Part model, mm, in its own coordinate system. Face numbers are marked on the shaded views. A direction names the side the tool comes from. Round coordinates to 2 decimals unless told otherwise and drop trailing zeros. Write each loop counter-clockwise with the first axis right and the second up, starting at its lowest first coordinate (ties: lowest second). Pieces come first, ordered by that corner, then holes. Notation, with made-up numbers: M -21.75,32 L 37.25,32 A28 ccw 37.25,63 Z; hole C 11,-0.5 d1. An arc over 180 degrees is marked long. Use a Markdown table: item, result. Add a question column.
1) Slice it at A-A on y = 13.5. Write the cut outline in (x, z), plus the area to 3 significant figures.
2) Wall check: probe 1 along X at (y, z) = (13.5, 5.8); probe 2 along X at (y, z) = (13.5, 3.3); probe 3 along X at (y, z) = (7.5, 5.75). Give the ranges that are in metal, low to high.
3) Slice it at D-D on y = 8.5. Write the cut outline in (x, z).
4) Slice it at C-C on z = 1. Write the cut outline in (x, y), plus the area to 3 significant figures.
5) Which spindle directions (+Z, -Z, +X, -X, +Y, -Y) get a long thin tool onto all of the face, cutting with end or side? Do the marked faces 4, 5, 6 and 7. Say none if no direction does.
6) Drop flat-ended pins along their axis: P1, Ø5, axis at x = -35.5, y = 6, coming from the +Z side; P2, Ø1, axis at x = -12.5, z = 2.5, coming from the +Y side; P3, Ø0.9, axis at y = 15, z = 1.5, coming from the -X side; P4, Ø3.5, axis at y = 17, z = 1, coming from the +X side. Give the stop position or say it passes through.
7) Two-plate mould, pull along Y, no slides. Class the marked faces 1, 2 and 3: released by +Y, released by -Y, zero draft, split by the parting line, or undercut.
```python
from build123d import *

# Parameters (mm, degrees)
ESQUISSE1_W             = 45
ESQUISSE1_H             = 23
BOSS_EXTRU_1_DEPTH      = 6
ENL_V_MAT_EXTRU_1_DEPTH = 3
CONG_1_R                = 6
ENL_V_MAT_EXTRU_3_DEPTH = 1.3
ESQUISSE7_W             = 45
ESQUISSE7_H             = 2
ENL_V_MAT_EXTRU_4_DEPTH = 2
ESQUISSE8_R             = 5.5
ESQUISSE8_W             = 10
ESQUISSE8_H             = 11.05
ESQUISSE8_H_2           = 4.3
ENL_V_MAT_EXTRU_5_DEPTH = 51.8920426
ESQUISSE9_W             = 11.5
ESQUISSE9_H             = 8.5
ENL_V_MAT_EXTRU_6_DEPTH = 4
BOSS_EXTRU_2_DEPTH      = 0.7
ESQUISSE12_R            = 3.7
ENL_V_MAT_EXTRU_8_DEPTH = 1


with BuildPart() as part:
    # Esquisse1 → Boss.-Extru.1 (new body)
    with BuildSketch(Plane.XY):
        with Locations((-22.5, 11.5)):
            Rectangle(ESQUISSE1_W, ESQUISSE1_H)
    extrude(amount=BOSS_EXTRU_1_DEPTH)

    # Esquisse2 → Enlèv. mat.-Extru.1 (cut)
    with BuildSketch(Plane(origin=(0, 0, 0), x_dir=(-1, 0, 0), z_dir=(0, 0, -1))):
        Polygon((0, 23), (1.25, 23), (1.25, 2.7), (43.75, 2.7), (43.75, 23), (45, 23), (45, 0), (0, 0), align=None)
    extrude(amount=-ENL_V_MAT_EXTRU_1_DEPTH, mode=Mode.SUBTRACT)

    # Congé1
    cong_1_edges = [part.edges().sort_by_distance(p)[0] for p in [
        (-22.5, 23, 0),
    ]]
    fillet(cong_1_edges, radius=CONG_1_R - 0.0001)  # a hair under: the kernel refuses the full size

    # Esquisse6 → Enlèv. mat.-Extru.3 (cut)
    with BuildSketch(Plane(origin=(0, 0, 0), x_dir=(0, 0, -1), z_dir=(1, 0, 0))):
        with BuildLine():
            Line((-3, 17), (-3, 23.616482957))
            Line((-3, 23.616482957), (-6, 23.616482957))
            Line((-6, 23.616482957), (-6, 20))
            ThreePointArc((-6, 20), (-3.878679656, 19.121320344), (-3, 17))
        make_face()
    enl_v_mat_extru_3 = extrude(amount=-ENL_V_MAT_EXTRU_3_DEPTH, mode=Mode.SUBTRACT)

    # Symétrie2: Enlèv. mat.-Extru.3 across plane
    add(enl_v_mat_extru_3.mirror(Plane.ZY.offset(22.5)), mode=Mode.SUBTRACT)

    # Esquisse7 → Enlèv. mat.-Extru.4 (cut)
    with BuildSketch(Plane.XY.offset(6)):
        with Locations((-22.5, 16.2)):
            Rectangle(ESQUISSE7_W, ESQUISSE7_H)
    extrude(amount=-ENL_V_MAT_EXTRU_4_DEPTH, mode=Mode.SUBTRACT)

    # Esquisse8 → Enlèv. mat.-Extru.5 (cut, through all)
    with BuildSketch(Plane.XY.offset(6)):
        with Locations(Location((-26, 13.5, 0), (0, 0, 18.004453))):
            Circle(ESQUISSE8_R)
        with Locations((-37.5, 10.425)):
            Rectangle(ESQUISSE8_W, ESQUISSE8_H)
        with Locations((-9, 13.55)):
            Rectangle(ESQUISSE8_W, ESQUISSE8_H_2)
    extrude(amount=-ENL_V_MAT_EXTRU_5_DEPTH, mode=Mode.SUBTRACT)

    # Esquisse9 → Enlèv. mat.-Extru.6 (cut)
    with BuildSketch(Plane(origin=(0, 0, 0), x_dir=(-1, 0, 0), z_dir=(0, 0, -1))):
        with Locations((9, 13.55)):
            Rectangle(ESQUISSE9_W, ESQUISSE9_H)
    extrude(amount=-ENL_V_MAT_EXTRU_6_DEPTH, mode=Mode.SUBTRACT)

    # Esquisse10 → Boss.-Extru.2 (add)
    with BuildSketch(Plane.XY.offset(6)):
        with BuildLine():
            Line((-30.06939799, 17.2), (-21.93060201, 17.2))
            ThreePointArc((-21.93060201, 17.2), (-26, 19), (-30.06939799, 17.2))
        make_face()
        with BuildLine():
            Line((-31.230678732, 15.2), (-20.769321268, 15.2))
            ThreePointArc((-20.769321268, 15.2), (-26, 8), (-31.230678732, 15.2))
        make_face()
    extrude(amount=-BOSS_EXTRU_2_DEPTH)

    # Esquisse12 → Enlèv. mat.-Extru.8 (cut)
    with BuildSketch(Plane.XY.offset(6)):
        with Locations((-26, 13.5)):
            Circle(ESQUISSE12_R)
    extrude(amount=-ENL_V_MAT_EXTRU_8_DEPTH, mode=Mode.SUBTRACT)


solid = part.part
```
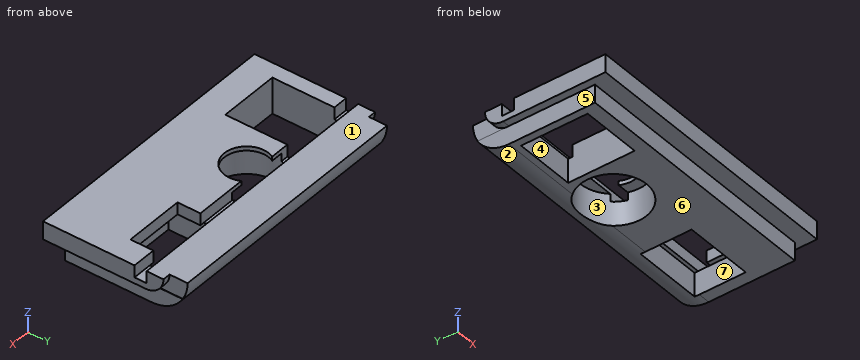
Entries:
| question | item | result |
|---|---|---|
| 1 | outline | M -45,3 L -43.75,3 L -43.75,0 L -42.5,0 L -42.5,6 L -45,6 Z; M -32.5,0 L -31.5,0 L -31.5,5.3 L -29.7,5.3 L -29.7,6 L -32.5,6 Z; M -22.3,5.3 L -20.5,5.3 L -20.5,0 L -14.75,0 L -14.75,4 L -14,4 L -14,6 L -22.3,6 Z; M -4,4 L -3.25,4 L -3.25,0 L -1.25,0 L -1.25,3 L 0,3 L 0,6 L -4,6 Z |
| 1 | area | 73.0 mm^2 |
| 2 | probe 1 | x = -45 to -42.5, -32.5 to -29.7, -22.3 to -14, -4 to 0 |
| 2 | probe 2 | x = -45 to -42.5, -32.5 to -31.5, -20.5 to -14.75, -3.25 to 0 |
| 2 | probe 3 | x = -45 to -42.5, -32.5 to 0 |
| 3 | outline | M -45,3 L -43.75,3 L -43.75,0 L -42.5,0 L -42.5,6 L -45,6 Z; M -32.5,0 L -28.29,0 L -28.29,5.3 L -23.71,5.3 L -23.71,0 L -1.25,0 L -1.25,3 L 0,3 L 0,6 L -32.5,6 Z |
| 4 | outline | M -43.75,2.7 L -1.25,2.7 L -1.25,20.32 L -43.75,20.32 Z; hole M -42.5,4.9 L -32.5,4.9 L -32.5,15.95 L -42.5,15.95 Z; hole C -26,13.5 d11; hole M -14.75,9.3 L -3.25,9.3 L -3.25,17.8 L -14.75,17.8 Z |
| 4 | area | 445 mm^2 |
| 5 | face 4 | +Z, -Z |
| 5 | face 5 | -Z, -X, +Y, -Y |
| 5 | face 6 | -Z, +X, -X, +Y, -Y |
| 5 | face 7 | -Z |
| 6 | P1 | stops at z = 6 |
| 6 | P2 | stops at y = 22.2 |
| 6 | P3 | stops at x = -43.75 |
| 6 | P4 | stops at x = -1.25 |
| 7 | face 1 | zero draft |
| 7 | face 2 | released by +Y |
| 7 | face 3 | undercut |
